Design review of the part shown in the three views and the two pictorial views. Dimensions are in mm from the part's minimum x, y and z. A direction names the side the tool comes from. Round coordinates to 2 decimals unless told otherwise and drop trailing zeros. Order: outer loops, then holes, each group sorted by start corner. A loop starts at its lowest first (then second) coordinate and runs counter-clockwise, first axis right, second up. Notation, with made-up numbers: M 81.25,58 L 122.25,58 A24 cw 122.25,77 Z; hole C 21.5,11 d4. An arc over 180 degrees is marked long. Use a Markdown table: item, result. Add a question column.
(1) To check wall thickness, follow probe 1 along Y at (x, z) = (31.75, 5.25) (3 decimals); probe 2 along X at (y, z) = (44, 9); probe 3 along Z at (x, y) = (6.5, 50.5). State the ranges of each line that lie inside material, in increasing order. Write a range as from..to.
(2) The part is to be moulded in two halves that separate along X. For the marked faces 3, 4, 5 and 6, say which applies: released by +X, released by -X, zero draft, split by the parting line, or undercut.
(3) For pin 1 (2 mm diameter, centred on x = 17, z = 13.5, fed in from +Y); pin 2 (8 mm diameter, centred on x = 41.5, y = 29.5, fed in from +Z), all flat-tipped, find the tip position at first contact; note any pin that passes through.
(4) Take a section at A-A (x = 31.75). Write out the cut boundary in (y, z) (3 decimals).
(5) Machinability: for the marked faces 1 and 2, which of the approach directions +Z, -Z, +X, -X, +Y, -Y give a long, thin tool a straight path to every point of the face, cutting with its end or side? Answer none if there is none.
(6) Take a section at B-B (y = 57.5). Write out the cut boundary in (x, z), then the cut area to 3 significant figures.
(7) Take a section at C-C (y = 34.5). Write out the cut boundary in (x, z).
(8) Take a section at D-D (x = 14.5). Write out the cut boundary in (y, z) (3 decimals), then the cut area to 3 significant figures.
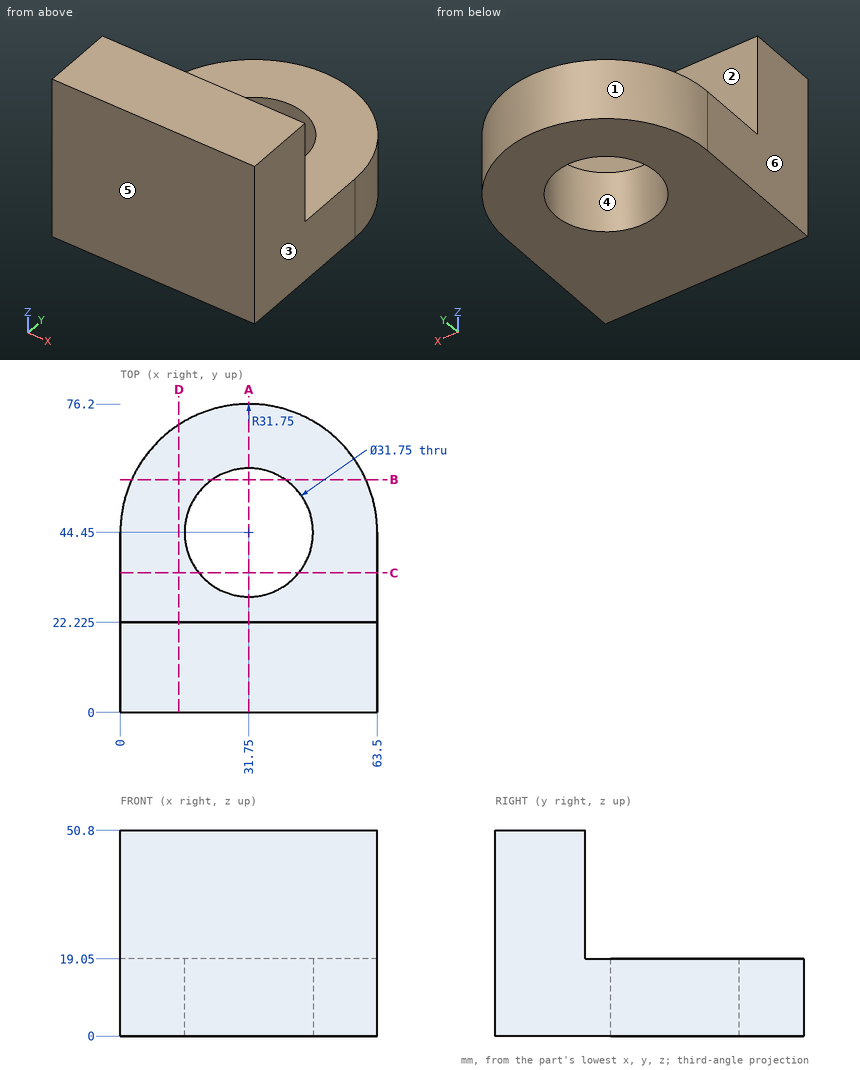
Verdict:
| question | item | result |
|---|---|---|
| 1 | probe 1 | y = 0..28.575, 60.325..76.2 |
| 1 | probe 2 | x = 0..15.88, 47.62..63.5 |
| 1 | probe 3 | z = 0..19.05 |
| 2 | face 3 | released by +X |
| 2 | face 4 | undercut |
| 2 | face 5 | zero draft |
| 2 | face 6 | released by -X |
| 3 | pin 1 | stops at y = 73.07 |
| 3 | pin 2 | stops at z = 19.05 |
| 4 | outline | M 0,0 L 28.575,0 L 28.575,19.05 L 22.225,19.05 L 22.225,50.8 L 0,50.8 Z; M 60.325,0 L 76.2,0 L 76.2,19.05 L 60.325,19.05 Z |
| 5 | face 1 | +Z, -Z, +Y |
| 5 | face 2 | +Z, +X, -X, +Y |
| 6 | outline | M 2.81,0 L 22.71,0 L 22.71,19.05 L 2.81,19.05 Z; M 40.79,0 L 60.69,0 L 60.69,19.05 L 40.79,19.05 Z |
| 6 | area | 758 mm^2 |
| 7 | outline | M 0,0 L 19.38,0 L 19.38,19.05 L 0,19.05 Z; M 44.12,0 L 63.5,0 L 63.5,19.05 L 44.12,19.05 Z |
| 8 | outline | M 0,0 L 71.105,0 L 71.105,19.05 L 22.225,19.05 L 22.225,50.8 L 0,50.8 Z |
| 8 | area | 2,060 mm^2 |
